from build123d import *

# Parameters (mm, degrees)
SKIZZE2_R                       = 1.6
AUFSATZ_LINEAR_AUSTRAGEN1_DEPTH = 5
SKIZZE3_R                       = 3
SCHNITT_LINEAR_AUSTRAGEN1_DEPTH = 2.5


with BuildPart() as part:
    # Skizze2 → Aufsatz-Linear austragen1 (new body)
    with BuildSketch(Plane(origin=(0, 0, 0), x_dir=(1, 0, 0), z_dir=(0, 1, 0))):
        with BuildLine():
            Line((-4, 28.5), (-4, -28.5))
            ThreePointArc((-4, -28.5), (1, -33.5), (6, -28.5))
            Line((6, -28.5), (6, 28.5))
            ThreePointArc((6, 28.5), (1, 33.5), (-4, 28.5))
        make_face()
        with Locations(Location((1, 28.5, 0), (0, 0, 270))):
            Circle(SKIZZE2_R, mode=Mode.SUBTRACT)
        with Locations(Location((1, 17.5, 0), (0, 0, 270))):
            Circle(SKIZZE2_R, mode=Mode.SUBTRACT)
        with Locations(Location((1, -17.5, 0), (0, 0, 90))):
            Circle(SKIZZE2_R, mode=Mode.SUBTRACT)
        with Locations(Location((1, -28.5, 0), (0, 0, 90))):
            Circle(SKIZZE2_R, mode=Mode.SUBTRACT)
    extrude(amount=AUFSATZ_LINEAR_AUSTRAGEN1_DEPTH)

    # Skizze3 → Schnitt-Linear austragen1 (cut)
    with BuildSketch(Plane.XZ):
        with Locations(Location((1, 17.5, 0), (0, 0, 270))):
            Circle(SKIZZE3_R)
        with Locations(Location((1, -17.5, 0), (0, 0, 270))):
            Circle(SKIZZE3_R)
    extrude(amount=-SCHNITT_LINEAR_AUSTRAGEN1_DEPTH, mode=Mode.SUBTRACT)


solid = part.part
The listing builds one solid part. Answer for the finished solid, in the listing's coordinates (mm). A direction names the side the tool comes from. Give positions to 0.01 mm unless a question says otherwise; leave off trailing zeros. Write each loop counter-clockwise with the first axis right and the second up, starting at its lowest first coordinate (ties: lowest second). Pieces come first, ordered by that corner, then holes.
Item 1: Find the intervals of material crossed by line 1 along X through (y, z) = (3.7, -17.5); line 2 along Z through (x, y) = (-0.75, 1.8); line 3 along Z through (x, y) = (0.5, 0.45), in increasing order.
Item 2: Section B-B, the plane x = 1 is taken. Write down the section's boundary in (y, z).
Item 3: Section A-A, the plane z = -17.5 is taken. Write down the section's boundary in (x, y), plus the area to 3 significant figures.
Item 4: Flat-ended cylindrical pins translate along their axes: P1, Ø3.5, axis at x = 1, z = 17.5, coming from the +Y side; P2, Ø1.8, axis at x = 2.5, z = -18.5, coming from the -Y side; P3, Ø1.9, axis at x = 1, z = 28.5, coming from the -Y side. Find the tip coordinate at first contact, or state that the pin passes through.
Item 5: Section D-D, the plane x = 5.25 is taken. Write down the section's boundary in (y, z), plus the area to 3 significant figures.
Item 6: Section C-C, the plane y = 1.55 is taken. Write down the section's boundary in (x, z), plus the area to 3 significant figures.
Item 7: Which of the six approach directions +Z, -Z, +X, -X, +Y, -Y give full straight-line access (tool end or side, diameter ignored) to faces 4 (the cylindrical face through (1.1, 1.2, 20.5)), 5 (the cylindrical face through (1.1, 2.5, -33.5))?
Item 8: Determine the mould class of faces 1 (the flat face through (1, 5, 0)), 2 (the flat face through (-4, 2, 0)), 3 (the cylindrical face through (-0.08, 2.46, 29.68)) for opening direction X: released by +X, released by -X, zero draft, split by the parting line, or undercut.
Completed:
1. line 1: x = -4 to -0.6, 2.6 to 6
1. line 2: z = -33.18 to -19.94, -15.06 to 15.06, 19.94 to 33.18
1. line 3: z = -33.47 to -30.02, -26.98 to -20.46, -14.54 to 14.54, 20.46 to 26.98, 30.02 to 33.47
2. outline: (0, -33.5) - (5, -33.5) - (5, -30.1) - (0, -30.1) - close; (0, -26.9) - (5, -26.9) - (5, -19.1) - (2.5, -19.1) - (2.5, -20.5) - (0, -20.5) - close; (0, -14.5) - (2.5, -14.5) - (2.5, -15.9) - (5, -15.9) - (5, 15.9) - (2.5, 15.9) - (2.5, 14.5) - (0, 14.5) - close; (0, 20.5) - (2.5, 20.5) - (2.5, 19.1) - (5, 19.1) - (5, 26.9) - (0, 26.9) - close; (0, 30.1) - (5, 30.1) - (5, 33.5) - (0, 33.5) - close
3. outline: (-4, 0) - (-2, 0) - (-2, 2.5) - (-0.6, 2.5) - (-0.6, 5) - (-4, 5) - close; (2.6, 2.5) - (4, 2.5) - (4, 0) - (6, 0) - (6, 5) - (2.6, 5) - close
3. area: 27.0 mm2
4. P1: stops at y = 5
4. P2: stops at y = 2.5
4. P3: passes through
5. outline: (0, -31.13) - (5, -31.13) - (5, 31.13) - (0, 31.13) - close
5. area: 311 mm2
6. outline: (-4, -28.5) arc R5 ccw to (6, -28.5) - (6, 28.5) arc R5 ccw to (-4, 28.5) - close; hole circle Ø6 at (1, -17.5); hole circle Ø6 at (1, 17.5); hole circle Ø3.2 at (1, -28.5); hole circle Ø3.2 at (1, 28.5)
6. area: 576 mm2
7. face 4: -Y
7. face 5: -Z, +Y, -Y
8. face 1: zero draft
8. face 2: released by -X
8. face 3: undercut
